from build123d import *

# Parameters (mm, degrees)
SKETCH1_W           = 724
SKETCH1_H           = 865
BOSS_EXTRUDE1_DEPTH = 1.27
SKETCH2_W           = 42
SKETCH2_H           = 135
SKETCH2_H_2         = 100
CUT_EXTRUDE1_DEPTH  = 1.27
SKETCH3_R           = 2.65
CUT_EXTRUDE2_DEPTH  = 1.27
LPATTERN1_COUNT     = 10
LPATTERN1_PITCH     = 78.222222222
FILLET1_R           = 5


with BuildPart() as part:
    # Sketch1 → Boss-Extrude1 (new body)
    with BuildSketch(Plane.XY):
        Rectangle(SKETCH1_W, SKETCH1_H)
    extrude(amount=BOSS_EXTRUDE1_DEPTH)

    # Sketch2 → Cut-Extrude1 (cut)
    with BuildSketch(Plane.XY.offset(1.27)):
        with Locations((-341, 175)):
            Rectangle(SKETCH2_W, SKETCH2_H)
        with Locations((-341, -332.5)):
            Rectangle(SKETCH2_W, SKETCH2_H_2)
        with Locations((341, 175)):
            Rectangle(SKETCH2_W, SKETCH2_H)
        with Locations((341, -332.5)):
            Rectangle(SKETCH2_W, SKETCH2_H_2)
    extrude(amount=-CUT_EXTRUDE1_DEPTH, mode=Mode.SUBTRACT)

    # Sketch3 → Cut-Extrude2 (cut)
    with BuildSketch(Plane.XY.offset(1.27)):
        with Locations((-352, 422.5)):
            Circle(SKETCH3_R)
        with Locations((-352, -422.5)):
            Circle(SKETCH3_R)
    cut_extrude2 = extrude(amount=-CUT_EXTRUDE2_DEPTH, mode=Mode.SUBTRACT)

    # LPattern1: Cut-Extrude2 ×10
    with Locations(*[(i * LPATTERN1_PITCH, 0, 0) for i in range(1, LPATTERN1_COUNT)]):
        add(cut_extrude2, mode=Mode.SUBTRACT)

    # Fillet1
    fillet1_edges = [part.edges().sort_by_distance(p)[0] for p in [
        (-362, -382.5, 0.635),
        (-362, -282.5, 0.635),
        (-320, -282.5, 0.635),
        (-320, -382.5, 0.635),
        (362, 242.5, 0.635),
        (362, 107.5, 0.635),
        (320, 107.5, 0.635),
        (320, 242.5, 0.635),
        (362, -282.5, 0.635),
        (362, -382.5, 0.635),
        (320, -382.5, 0.635),
        (320, -282.5, 0.635),
        (-362, 107.5, 0.635),
        (-362, 242.5, 0.635),
        (-320, 242.5, 0.635),
        (-320, 107.5, 0.635),
        (-362, 432.5, 0.635),
        (362, 432.5, 0.635),
        (362, -432.5, 0.635),
        (-362, -432.5, 0.635),
    ]]
    fillet(fillet1_edges, radius=FILLET1_R)


solid = part.part
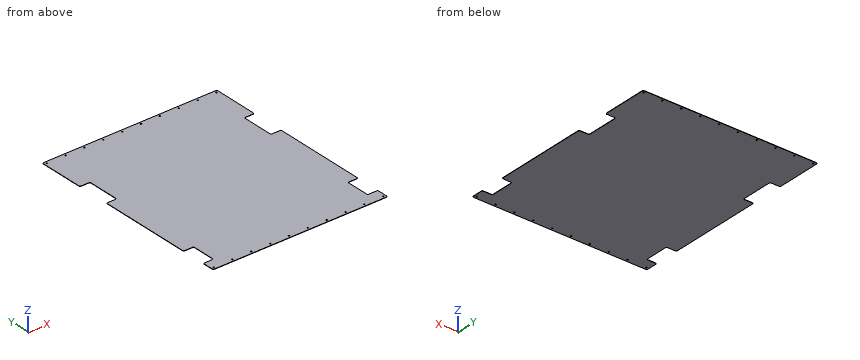
CAD build for the part. Positions are in the model's coordinates, mm. Coordinates: 2 decimals unless noted, no trailing zeros. Answer as a JSON object with one key per item and string values. Group by question number.
1) Pin check, flat tips, straight feed: pin 1 Ø4 at (x, y) = (39.11, 422.5) entering from -Z; pin 2 Ø0.6 at (y, z) = (-316, 1) entering from +X. Stop position of each tip, or through.
2) Wall check: line 1 (Y direction, x = -352, z = 0.9); line 2 (Y direction, x = 321, z = 0.4); line 3 (X direction, y = -349, z = 0.9). Give the ranges that are in metal, low to high. Write a range as from..to.
3) Saw through at A-A (z = 0.5). Give the number of separate pieces and of enclosed holes in the cut face, plus the area to 3 significant figures.
Values follow:
{
 "1": {"pin 1": "passes through", "pin 2": "stops at x = 320"},
 "2": {"line 1": "y = -432.5..-425.15, -419.85..-382.5, -282.5..107.5, 242.5..419.85, 425.15..432.5", "line 2": "y = -432.5..-380.5, -284.5..109.5, 240.5..432.5", "line 3": "x = -320..320"},
 "3": {"separate pieces": "1", "enclosed holes": "20", "area": "606,000 mm2"}
}
